Autodesk Inventor part; units mm, degrees
ref_plane "Start Plane" through (0, 0, 0) normal (0, 0, 1) x (1, 0, 0)
ref_plane "End Plane" through (0, 0, 200) normal (0, 0, 1) x (1, 0, 0)
ref_plane "YZ Plane" through (0, 0, 0) normal (1, 0, 0) x (0, 1, 0)
ref_plane "Start Plane" through (0, 0, 0) normal (0, 0, 1) x (1, 0, 0)
ref_plane "End Plane" through (0, 0, 200) normal (0, 0, 1) x (1, 0, 0)
sketch "Sketch" plane through (0, 0, 0) normal (0, 0, 1) x (1, 0, 0)
  circle A0 centre (0, 0) radius 2.5
  circle A1 centre (0, 0) radius 4.2 construction
  line L0 (10, -10) -> (-10, -10) construction
  line L1 (-10, -10) -> (-10, 10) construction
  line L2 (-10, 10) -> (10, 10) construction
  line L3 (10, 10) -> (10, -10) construction
  line L4 (10, -10) -> (-10, 10) construction
  line L5 (-10, -10) -> (10, 10) construction
  line L6 (-4.1658, 3.1759) -> (-7.7464, 6.7565)
  line L7 (-10, 8.8) -> (-10, 3.95)
  line L8 (-10, 3.95) -> (-9.6, 3.95)
  line L9 (-9.6, 3.95) -> (-9.6, 3.2)
  line L10 (-9.6, 3.2) -> (-8.6, 3.2)
  line L11 (-8.6, 3.2) -> (-8.6, 6.4029)
  line L12 (-10, 0) -> (0, 0) construction
  line L13 (-8.8, 10) -> (-3.95, 10)
  line L14 (-3.95, 10) -> (-3.95, 9.6)
  line L15 (-3.95, 9.6) -> (-3.2, 9.6)
  line L16 (-3.2, 9.6) -> (-3.2, 8.6)
  line L17 (-3.2, 8.6) -> (-6.4029, 8.6)
  arc A2 (-8.8, 10) -> (-10, 8.8) centre (-8.8, 8.8) ccw
  arc A3 (-6.4029, 8.6) -> (-6.7565, 7.7464) centre (-6.4029, 8.1) ccw
  arc A4 (-7.7464, 6.7565) -> (-8.6, 6.4029) centre (-8.1, 6.4029) ccw
  arc A5 (-3.8668, 1.6394) -> (-4.2, 0) centre (0, 0) ccw
  arc A6 (-3.8668, 1.6394) -> (-4.1658, 3.1759) centre (-5.1558, 2.1859) ccw
  line L18 (-3.1759, 4.1658) -> (-6.7565, 7.7464)
  arc A7 (0, 4.2) -> (-1.6394, 3.8668) centre (0, 0) ccw
  arc A8 (-3.1759, 4.1658) -> (-1.6394, 3.8668) centre (-2.1859, 5.1558) ccw
  line L19 (-3.2, -9.6) -> (-3.2, -8.6)
  line L20 (-3.2, -8.6) -> (-6.4029, -8.6)
  line L21 (-8.8, -10) -> (-3.95, -10)
  arc A9 (-1.6394, -3.8668) -> (-3.1759, -4.1658) centre (-2.1859, -5.1558) ccw
  line L22 (-3.1759, -4.1658) -> (-6.7565, -7.7464)
  line L23 (0, -10) -> (0, 0) construction
  arc A10 (-4.1658, -3.1759) -> (-3.8668, -1.6394) centre (-5.1558, -2.1859) ccw
  line L24 (-4.1658, -3.1759) -> (-7.7464, -6.7565)
  line L25 (-3.95, -9.6) -> (-3.2, -9.6)
  line L26 (-3.95, -10) -> (-3.95, -9.6)
  arc A11 (-1.6394, -3.8668) -> (0, -4.2) centre (0, 0) ccw
  arc A12 (-4.2, 0) -> (-3.8668, -1.6394) centre (0, 0) ccw
  line L27 (-9.6, -3.95) -> (-9.6, -3.2)
  arc A13 (-6.7565, -7.7464) -> (-6.4029, -8.6) centre (-6.4029, -8.1) ccw
  arc A14 (-8.6, -6.4029) -> (-7.7464, -6.7565) centre (-8.1, -6.4029) ccw
  line L28 (-8.6, -3.2) -> (-8.6, -6.4029)
  line L29 (-9.6, -3.2) -> (-8.6, -3.2)
  line L30 (-10, -3.95) -> (-9.6, -3.95)
  line L31 (-10, -8.8) -> (-10, -3.95)
  arc A15 (-10, -8.8) -> (-8.8, -10) centre (-8.8, -8.8) ccw
  line L32 (9.6, -3.2) -> (8.6, -3.2)
  line L33 (8.6, -3.2) -> (8.6, -6.4029)
  line L34 (10, -8.8) -> (10, -3.95)
  arc A16 (3.8668, -1.6394) -> (4.1658, -3.1759) centre (5.1558, -2.1859) ccw
  line L35 (4.1658, -3.1759) -> (7.7464, -6.7565)
  line L36 (10, 0) -> (0, 0) construction
  arc A17 (3.1759, -4.1658) -> (1.6394, -3.8668) centre (2.1859, -5.1558) ccw
  line L37 (3.1759, -4.1658) -> (6.7565, -7.7464)
  line L38 (9.6, -3.95) -> (9.6, -3.2)
  line L39 (10, -3.95) -> (9.6, -3.95)
  arc A18 (3.8668, -1.6394) -> (4.2, 0) centre (0, 0) ccw
  arc A19 (0, -4.2) -> (1.6394, -3.8668) centre (0, 0) ccw
  line L40 (3.95, -9.6) -> (3.2, -9.6)
  arc A20 (7.7464, -6.7565) -> (8.6, -6.4029) centre (8.1, -6.4029) ccw
  arc A21 (6.4029, -8.6) -> (6.7565, -7.7464) centre (6.4029, -8.1) ccw
  line L41 (3.2, -8.6) -> (6.4029, -8.6)
  line L42 (3.2, -9.6) -> (3.2, -8.6)
  line L43 (3.95, -10) -> (3.95, -9.6)
  line L44 (8.8, -10) -> (3.95, -10)
  arc A22 (8.8, -10) -> (10, -8.8) centre (8.8, -8.8) ccw
  line L45 (3.2, 9.6) -> (3.2, 8.6)
  line L46 (3.2, 8.6) -> (6.4029, 8.6)
  line L47 (8.8, 10) -> (3.95, 10)
  arc A23 (1.6394, 3.8668) -> (3.1759, 4.1658) centre (2.1859, 5.1558) ccw
  line L48 (3.1759, 4.1658) -> (6.7565, 7.7464)
  line L49 (0, 10) -> (0, 0) construction
  arc A24 (4.1658, 3.1759) -> (3.8668, 1.6394) centre (5.1558, 2.1859) ccw
  line L50 (4.1658, 3.1759) -> (7.7464, 6.7565)
  line L51 (3.95, 9.6) -> (3.2, 9.6)
  line L52 (3.95, 10) -> (3.95, 9.6)
  arc A25 (1.6394, 3.8668) -> (0, 4.2) centre (0, 0) ccw
  arc A26 (4.2, 0) -> (3.8668, 1.6394) centre (0, 0) ccw
  line L53 (9.6, 3.95) -> (9.6, 3.2)
  arc A27 (6.7565, 7.7464) -> (6.4029, 8.6) centre (6.4029, 8.1) ccw
  arc A28 (8.6, 6.4029) -> (7.7464, 6.7565) centre (8.1, 6.4029) ccw
  line L54 (8.6, 3.2) -> (8.6, 6.4029)
  line L55 (9.6, 3.2) -> (8.6, 3.2)
  line L56 (10, 3.95) -> (9.6, 3.95)
  line L57 (10, 8.8) -> (10, 3.95)
  arc A29 (10, 8.8) -> (8.8, 10) centre (8.8, 8.8) ccw
  point P0 (-3.4233, 2.4333)
  point P1 (-8.6, 7.6101)
  point P2 (-7.6101, 8.6)
  point P3 (-7.6101, -8.6)
  point P4 (-10, -10)
  point P5 (-2.4333, -3.4233)
  point P6 (-8.6, -7.6101)
  point P7 (8.6, -7.6101)
  point P8 (10, -10)
  point P9 (3.4233, -2.4333)
  point P10 (7.6101, -8.6)
  point P11 (7.6101, 8.6)
  point P12 (10, 10)
  point P13 (2.4333, 3.4233)
  point P14 (8.6, 7.6101)
  point P15 (-4.2, 0)
  point P16 (0, -4.2)
  point P17 (4.2, 0)
  point P18 (0, 4.2)
  dimension "d8" = 5
  dimension "d9" = 8.4
  dimension "d10" = 20
  dimension "d11" = 20
  dimension "d13" = 1.4
  dimension "d14" = 3.2
  dimension "d15" = 3.95
  dimension "d16" = 0.4
  dimension "d18" = 1.2
  dimension "d19" = 0.5
  dimension "d20" = 1.4
  dimension "d21" = 1.4
  dimension "d24" = 360
extrude "Body" add sketch "Sketch" along normal up to surface (200 mm away) from surface at 0
sketch "Sketch11" plane through (0, 0, 0) normal (0, 0, 1) x (1, 0, 0)
  line L0 (0, 0) -> (10, 0)
ref_plane "Work Plane11" through (0, 0, 0) normal (0, -1, 0) x (1, 0, 0)
sketch "Sketch12" plane through (0, 0, 0) normal (0, -1, 0) x (1, 0, 0)
  line L0 (-2, 0) -> (12, 0)
  line L1 (-2, 200) -> (12, 200)
  dimension "d53" = 200
equation "\"G_OFFSET_START\" = 0"
equation "\"G_OFFSET_END\" = 0"
equation "\"G_L\" = d53"
equation "\"G_OFFSET_START1\" = 0"
equation "\"G_OFFSET_END1\" = 0"
equation "\"G_OFFSET_START2\" = 0"
equation "\"G_OFFSET_END2\" = 0"
properties part number "2020Profile" material "Aluminum 6061"
Part model, mm, in its own coordinate system. A direction names the side the tool comes from. Round coordinates to 2 decimals unless told otherwise and drop trailing zeros. Return JSON: item names as keys, results as strings. Group by question number.
(1) Pin check, flat tips, straight feed: pin 1 Ø0.8 at (x, z) = (-3.5, 63) entering from -Y; pin 2 Ø0.8 at (x, z) = (-9, 120) entering from +Y; pin 3 Ø2 at (x, y) = (-4.5, 7) entering from -Z; pin 4 Ø0.8 at (y, z) = (-3.5, 130) entering from -X. Stop position of each tip, or through.
(2) Two-plate mould, pull along X, no slides. Class faces 1 (the face through (-5, 8.6, 99)), 2 (the face through (2, 2, 200)), 3 (the face through (10, 6, 99)): +X half, -X half, draft (parallel to the pull), parting line (faces both ways), or undercut.
(3) Which spindle directions (+Z, -Z, +X, -X, +Y, -Y) get a long thin tool onto all of the face, cutting with end or side? Do faces 4 (the face through (4.94, 5.93, 98.6)), 5 (the face through (-6, -10, 99)). Say none if no direction does.
(4) Drill centre lines: probe 1 along Y at (x, z) = (0, 114); probe 2 along X at (y, z) = (-3.5, 175); probe 3 along X at (y, z) = (6, 55.5). Where is each one in solid material? Low to high.
Returned:
{
 "1": {"pin 1": "y = -9.6", "pin 2": "y = 10", "pin 3": "through", "pin 4": "x = -9.6"},
 "2": {"face 1": "undercut", "face 2": "draft", "face 3": "+X half"},
 "3": {"face 4": "+Z, -Z", "face 5": "+Z, -Z, +X, -X, -Y"},
 "4": {"probe 1": "-4.2 to -2.5, 2.5 to 4.2", "probe 2": "-9.6 to -8.6, -4.49 to 4.49, 8.6 to 9.6", "probe 3": "-10 to -8.6, -6.99 to -5.01, 5.01 to 6.99, 8.6 to 10"}
}
